Here's how the part is built. I have some questions about the finished solid (model axes, mm). Face numbers are marked on the shaded views. A direction names the side the tool comes from. Coordinates: 2 decimals unless noted, no trailing zeros. Write each loop counter-clockwise with the first axis right and the second up, starting at its lowest first coordinate (ties: lowest second). Pieces come first, ordered by that corner, then holes.
Item 1: I want a section at B-B (z = 21.5). Please give me the cut outline in (x, y), and give its area (3 significant figures).
Item 2: I want a section at A-A (y = 0). Please give me the cut outline in (x, z), and give its area (3 significant figures).
Item 3: I want a section at C-C (z = 5). Please give me the cut outline in (x, y).
Item 4: I'm going to push flat-ended pins straight in: P1, Ø3.5, axis at y = 0, z = 21.5, coming from the +X side; P2, Ø6, axis at x = 0.5, z = 15.5, coming from the +Y side; P3, Ø6, axis at y = 2.5, z = 11, coming from the -X side. Where does each tip first touch, or does it pass through?
Item 5: For the marked faces 1 and 2, which set-ups out of +Z, -Z, +X, -X, +Y, -Y let a thin tool reach every point of the face, with its end or its side?
Item 6: Please list where these lines run through material, in increasing order: line 1 (Z direction, x = -3.8, y = 0); line 2 (Y direction, x = -1.5, z = 21.5); line 3 (Z direction, x = -4.5, y = 1).
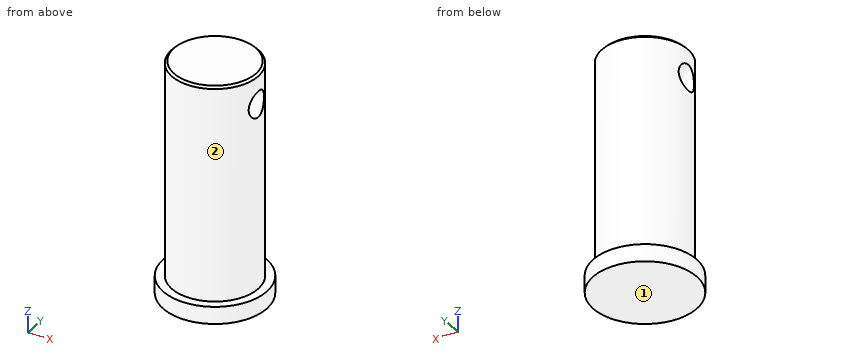
Solid Edge part; units mm, degrees
sketch "Sketch1" plane through (0, 0, 0) normal (0, 0, 1) x (1, 0, 0)
  circle A0 centre (0, 0) radius 5
extrude "Protrusion1" add sketch "Sketch1" along normal blind 25
sketch "Sketch2" plane through (0, 0, 0) normal (0, 0, -1) x (1, 0, 0)
  circle A0 centre (0, 0) radius 6
extrude "Protrusion2" add sketch "Sketch2" along normal blind 2
hole "Hole1" at (0, 0, 21.5) direction (1, 0, 0) diameter 3 end through all both ways yes
chamfer "Chamfer1" distance 0.25 angle 45 1 edges at (-5, 0, 25)
properties part number "87451"
Answer:
1. outline: (-4.77, -1.5) arc R5 ccw to (4.77, -1.5) - close; (-4.77, 1.5) - (4.77, 1.5) arc R5 ccw to start
1. area: 49.0 mm2
2. outline: (-6, -2) - (6, -2) - (6, 0) - (5, 0) - (5, 20) - (-5, 20) - (-5, 0) - (-6, 0) - close; (-5, 23) - (5, 23) - (5, 24.75) - (4.75, 25) - (-4.75, 25) - (-5, 24.75) - close
2. area: 244 mm2
3. outline: circle Ø10 at (0, 0)
4. P1: stops at x = 5
4. P2: stops at y = 5
4. P3: stops at x = -5
5. face 1: -Z, +X, -X, +Y, -Y
5. face 2: +Z
6. line 1: z = -2 to 20, 23 to 25
6. line 2: y = -4.77 to -1.5, 1.5 to 4.77
6. line 3: z = -2 to 20.38, 22.62 to 25
